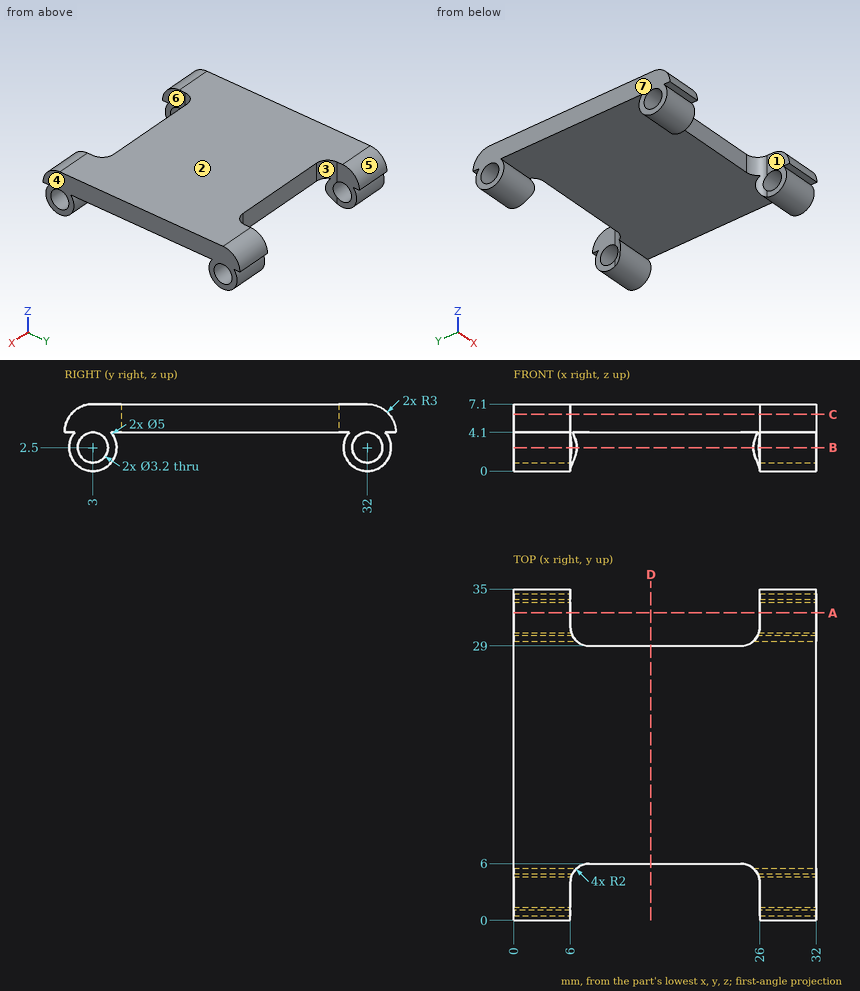
Verification items for this drawing (mm, ordinates from the low corner). A direction names the side the tool comes from. Coordinates: 2 decimals unless noted, no trailing zeros. Loops run counter-clockwise (first coordinate to the right, second up) from the corner with the lowest first, then second, coordinate; pieces in that order, holes last.
Item 1: Sectioned sample at D-D, the plane x = 14.5. Record the boundary of the cut face in (y, z), then the cut area to 3 significant figures.
Item 2: Sectioned sample at C-C, the plane z = 6. Record the boundary of the cut face in (x, y).
Item 3: Thickness scan on line 1 (Y direction, x = 29.25, z = 2.5); line 2 (Z direction, x = 29.5, y = 32); line 3 (Z direction, x = 4, y = 24). Record the ranges inside material, lowest first.
Item 4: Sectioned sample at A-A, the plane y = 32.5. Record the boundary of the cut face in (x, z), then the cut area to 3 significant figures.
Item 5: Go/stop test with flat-tipped pins: pin 1 Ø2 at (x, y) = (6.5, 17.5) entering from -Z; pin 2 Ø1.2 at (x, y) = (30, 0.5) entering from -Z (1 decimal); pin 3 Ø3.5 at (x, z) = (16, 6) entering from +Y; pin 4 Ø3 at (y, z) = (1.5, 2.5) entering from +X. Record where each tip stops, or that it passes through.
Item 6: Sectioned sample at B-B, the plane z = 2.5. Count the separate pieces of the cut face and the enclosed holes in it, then the cut area to 3 significant figures.
Item 7: Release check for a two-part mould opening along X. For the marked faces 4, 5, 6 and 7 record: released by +X, released by -X, zero draft, split by the parting line, or undercut.
Item 8: Access from +Z, -Z, +X, -X, +Y, -Y to the whole of each face (thin tool, end or side, straight path). Record for the marked faces 1, 2 and 3.
Check result:
1. outline: (6, 4.1) - (29, 4.1) - (29, 7.1) - (6, 7.1) - close
1. area: 69.0 mm2
2. outline: (0, 0.68) - (6, 0.68) - (6, 4) arc R2 cw to (8, 6) - (24, 6) arc R2 cw to (26, 4) - (26, 0.68) - (32, 0.68) - (32, 34.32) - (26, 34.32) - (26, 31) arc R2 cw to (24, 29) - (8, 29) arc R2 cw to (6, 31) - (6, 34.32) - (0, 34.32) - close
3. line 1: y = 0.5 to 1.4, 4.6 to 5.5, 29.5 to 30.4, 33.6 to 34.5
3. line 2: z = 0 to 0.9, 4.1 to 7.1
3. line 3: z = 4.1 to 7.1
4. outline: (0, 0.05) - (6, 0.05) - (6, 0.98) - (0, 0.98) - close; (0, 4.02) - (6, 4.02) - (6, 7.06) - (0, 7.06) - close; (26, 0.05) - (32, 0.05) - (32, 0.98) - (26, 0.98) - close; (26, 4.02) - (32, 4.02) - (32, 7.06) - (26, 7.06) - close
4. area: 47.6 mm2
5. pin 1: stops at z = 4.1
5. pin 2: stops at z = 0.9
5. pin 3: stops at y = 29
5. pin 4: stops at x = 32
6. separate pieces: 8
6. enclosed holes: 0
6. area: 44.4 mm2
7. face 4: released by +X
7. face 5: zero draft
7. face 6: undercut
7. face 7: released by -X
8. face 1: +Z, -Z, -Y
8. face 2: +Z, +X, -X, +Y, -Y
8. face 3: +Z, -Z, +Y
